```python
from build123d import *

# Parameters (mm, degrees)
Y_KSEKLIK_EKSTR_ZYON1_DEPTH = 12
IZIM3_R                     = 5
Y_KSEKLIK_EKSTR_ZYON3_DEPTH = 7
IZIM2_R                     = 2.701874654
IZIM2_R_2                   = 1.49
Y_KSEKLIK_EKSTR_ZYON2_DEPTH = 8


with BuildPart() as part:
    # Çizim1 → Yükseklik-Ekstrüzyon1 (new body)
    with BuildSketch(Plane.XY):
        with BuildLine():
            Line((4.73249152, 1.451214667), (6.9, 1.451214667))
            Line((6.9, 1.451214667), (6.9, -1.398785333))
            Line((6.9, -1.398785333), (4.748252267, -1.398785333))
            ThreePointArc((4.748252267, -1.398785333), (0, -4.95), (-4.748252267, -1.398785333))
            Line((-4.748252267, -1.398785333), (-6.9, -1.398785333))
            Line((-6.9, -1.398785333), (-6.9, 1.451214667))
            Line((-6.9, 1.451214667), (-4.73249152, 1.451214667))
            ThreePointArc((-4.73249152, 1.451214667), (0, 4.95), (4.73249152, 1.451214667))
        make_face()
        with BuildLine():
            Line((1.523723566, -2.106719368), (-1.523723566, -2.106719368))
            ThreePointArc((-1.523723566, -2.106719368), (0, 2.6), (1.523723566, -2.106719368))
        make_face(mode=Mode.SUBTRACT)
    extrude(amount=Y_KSEKLIK_EKSTR_ZYON1_DEPTH)

    # Çizim3 → Yükseklik-Ekstrüzyon3 (add)
    with BuildSketch(Plane.XY.offset(12)):
        with Locations(Location((0, 0, 0), (0, 0, 196.245706225))):
            Circle(IZIM3_R)
        with BuildLine():
            Line((-1.523723566, -2.106719368), (1.523723566, -2.106719368))
            ThreePointArc((1.523723566, -2.106719368), (0, 2.6), (-1.523723566, -2.106719368))
        make_face(mode=Mode.SUBTRACT)
    extrude(amount=Y_KSEKLIK_EKSTR_ZYON3_DEPTH)

    # Çizim2 → Yükseklik-Ekstrüzyon2 (add)
    with BuildSketch(Plane.XY):
        Circle(IZIM2_R)
        Circle(IZIM2_R_2, mode=Mode.SUBTRACT)
    extrude(amount=Y_KSEKLIK_EKSTR_ZYON2_DEPTH)


solid = part.part
```
Could you check a few things on this model? Use its own coordinates, in mm. A direction names the side the tool comes from. Round coordinates to 2 decimals unless told otherwise and drop trailing zeros. Loops run counter-clockwise (first coordinate to the right, second up) from the corner with the lowest first, then second, coordinate; pieces in that order, holes last. Notation, with made-up numbers: M 17.25,4.25 L 46.25,4.25 A16 ccw 46.25,27.25 Z; hole C -27.75,53 d4. An arc over 180 degrees is marked long. Put each result on its own line as item: value.
Q1. For pin 1 (0.6 mm diameter, centred on x = 6, y = -0.5, fed in from +Z); pin 2 (1.7 mm diameter, centred on x = -6, z = 4.5, fed in from -Y); pin 3 (2 mm diameter, centred on x = -1.5, z = 7, fed in from -Y), each with a flat end and sliding along its axis, tell me the tip position at first contact or that it passes through.
Check result:
pin 1: z = 12
pin 2: y = -1.4
pin 3: y = -4.92
Q2. Imagine slicing it at D-D (x = 2.25). Write out the boundary of the cut face in (y, z).
Check result:
outline: M -4.47,12 L -4.41,12 L -4.41,0 L 4.41,0 L 4.41,12 L 4.47,12 L 4.47,19 L 1.3,19 L 1.3,8 L -1.3,8 L -1.3,19 L -4.47,19 Z
Q3. On a 3-axis mill with a long thin cutter (end or side, diameter ignored), from which of +Z, -Z, +X, -X, +Y, -Y can I reach the whole of each face in a straight line? I mean faces 5 (the face through (6.9, 0, 6)), 6 (the face through (0, -2.107, 13)), 7 (the face through (0.09, -4.95, 5.92)). Say none if no direction works.
Check result:
face 5: +Z, -Z, +X, +Y, -Y
face 6: +Z
face 7: -Z, -Y
Q4. Thinking about a two-plate mould opening in Y: for faces 1 (the face through (-0.194, 1.477, 3.944)), 2 (the face through (-0.09, 4.95, 5.92)), 3 (the face through (-1.2, 1.3, 8)), 4 (the face through (-6, -1.399, 6)), which applies, released by +Y, released by -Y, zero draft, split by the parting line, or undercut?
Check result:
face 1: undercut
face 2: released by +Y
face 3: undercut
face 4: released by -Y
Q5. Imagine slicing it at C-C (y = 1). Write out the boundary of the cut face in (x, z).
Check result:
outline: M -6.9,0 L -1.1,0 L -1.1,8 L -2.4,8 L -2.4,19 L -4.9,19 L -4.9,12 L -6.9,12 Z; M 1.1,0 L 6.9,0 L 6.9,12 L 4.9,12 L 4.9,19 L 2.4,19 L 2.4,8 L 1.1,8 Z
Q6. I need wall thicknesses on probe 1 along X at (y, z) = (0, 9.2); probe 2 along Y at (x, z) = (0, 14.25); probe 3 along X at (y, z) = (0, 16.5). Which ranges of each line are inside material? Lowest first, please.
Check result:
probe 1: -6.9 to -2.6, 2.6 to 6.9
probe 2: -5 to -2.11, 2.6 to 5
probe 3: -5 to -2.6, 2.6 to 5
Q7. Imagine slicing it at A-A (x = 0). Write out the boundary of the cut face in (y, z).
Check result:
outline: M -5,12 L -4.95,12 L -4.95,0 L -1.49,0 L -1.49,8 L -2.11,8 L -2.11,19 L -5,19 Z; M 1.49,0 L 4.95,0 L 4.95,12 L 5,12 L 5,19 L 2.6,19 L 2.6,8 L 1.49,8 Z
Q8. Imagine slicing it at B-B (z = 9.25). Write out the boundary of the cut face in (x, y).
Check result:
outline: M -6.9,-1.4 L -4.75,-1.4 A4.95 ccw 4.75,-1.4 L 6.9,-1.4 L 6.9,1.45 L 4.73,1.45 A4.95 ccw -4.73,1.45 L -6.9,1.45 Z; hole M -1.52,-2.11 L 1.52,-2.11 A2.6 ccw long Z
